Work out the finished part from the listing and answer in its coordinate system (mm). Face numbers are marked on the shaded views. A direction names the side the tool comes from. Round coordinates to 2 decimals unless told otherwise and drop trailing zeros. Order: outer loops, then holes, each group sorted by start corner. A loop starts at its lowest first (then second) coordinate and runs counter-clockwise, first axis right, second up. Notation, with made-up numbers: (30, -13.5) - (40, -13.5) arc R8 ccw to (40, 0.5) - close; hole circle Ø2 at (-18, 38). An arc over 180 degrees is marked (long way). One line per question, with ' | ' between items. Start each with the question number.
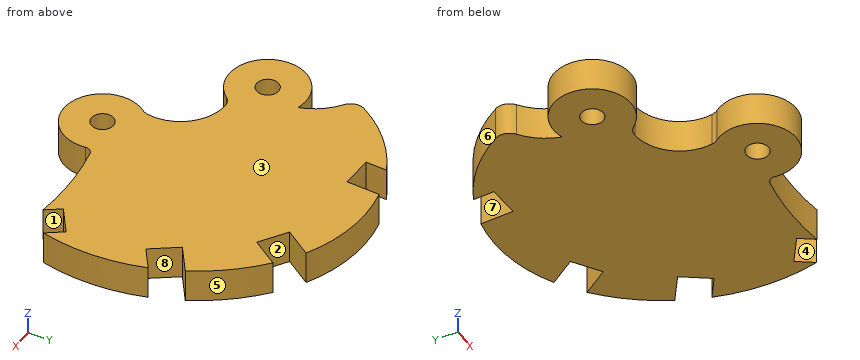
from build123d import *

# Parameters (mm, degrees)
SKETCH_1_R          = 1
EXTRUDE_1_DEPTH     = 3
CUT_EXTRUDE_1_DEPTH = 3
FILLET_3_R          = 0.635
FILLET_4_R          = 1.27
FILLET_5_R          = 1.27


with BuildPart() as part:
    # 스케치1 → 보스-돌출1 (new body)
    with BuildSketch(Plane.XY):
        with BuildLine():
            ThreePointArc((13.953884727, -10.4604054), (14.378598245, 0.342544853), (8.460782986, 9.390394228))
            ThreePointArc((8.460782986, 9.390394228), (-2.974719352, 12.059159282), (-12.129056489, 4.704491905))
            ThreePointArc((-12.129056489, 4.704491905), (-10.212753099, 3.28852822), (-9.098885827, 1.182234902))
            ThreePointArc((-9.098885827, 1.182234902), (-13.440703993, -3.372455138), (-7.178058569, -3.985528264))
            ThreePointArc((-7.178058569, -3.985528264), (-3.531014476, -5.328655626), (-2.617256463, -9.106216747))
            ThreePointArc((-2.617256463, -9.106216747), (-0.772979034, -14.843576338), (3.363017442, -10.4604054))
            ThreePointArc((3.363017442, -10.4604054), (8.658451084, -9.881913195), (13.953884727, -10.4604054))
        make_face()
        with Locations((-10.16, -2.153036707)):
            Circle(SKETCH_1_R, mode=Mode.SUBTRACT)
        with Locations((0, -11.43)):
            Circle(SKETCH_1_R, mode=Mode.SUBTRACT)
    extrude(amount=EXTRUDE_1_DEPTH)

    # 스케치2 → 컷-돌출1 (cut)
    with BuildSketch(Plane.XY.offset(3)):
        Polygon((12.294266072, -0.611273139), (10.692062425, 1.799944079), (13.190733117, 3.460258739), (14.792936764, 1.049041521), align=None)
        Polygon((-5.738219006, 9.252553702), (-2.846256152, 9.119979742), (-2.708873811, 12.11683244), (-5.600836664, 12.2494064), align=None)
        Polygon((4.882638145, 8.263381657), (7.266602202, 6.620901711), (8.96865396, 9.091330786), (6.584689903, 10.733810732), align=None)
        Polygon((11.087961457, -8.762836531), (13.499178676, -7.160632884), (15.159493336, -9.659303577), (12.748276117, -11.261507224), align=None)
    extrude(amount=-CUT_EXTRUDE_1_DEPTH, mode=Mode.SUBTRACT)

    # 필렛3
    fillet_3_edges = [part.edges().sort_by_distance(p)[0] for p in [
        (3.363017442, -10.4604054, 1.5),
    ]]
    fillet(fillet_3_edges, radius=FILLET_3_R)

    # 필렛4
    fillet_4_edges = [part.edges().sort_by_distance(p)[0] for p in [
        (-12.129056489, 4.704491905, 1.5),
    ]]
    fillet(fillet_4_edges, radius=FILLET_4_R)

    # 필렛5
    fillet_5_edges = [part.edges().sort_by_distance(p)[0] for p in [
        (-2.617256463, -9.106216747, 1.5),
        (-7.178058569, -3.985528264, 1.5),
    ]]
    fillet(fillet_5_edges, radius=FILLET_5_R)


solid = part.part
1) Section B-B on y = -11.43 is taken. Give the vertices of the cut face in (x, z), and give its area (3 significant figures).
2) For the marked faces 4, 5, 6, 7 and 8, determine the directions among +Z, -Z, +X, -X, +Y, -Y from which every point of the face is accessible in a straight line to the end or side of a thin tool.
3) Determine the mould class of the marked faces 1, 2 and 3 for opening direction X: released by +X, released by -X, zero draft, split by the parting line, or undercut.
4) Section C-C on x = -10.16 is taken. Give the vertices of the cut face in (y, z).
5) Section D-D on z = 1.1 is taken. Give the number of separate pieces and of enclosed holes in the cut face, and give its area (3 significant figures).
6) Straight lines are drawn through the part: line 1 (Y direction, x = -10.25, z = 2.35); line 2 (Y direction, x = -10.16, z = 1.1); line 3 (Y direction, x = 0, z = 0.95). For each, find the intervals that lie inside material, in ascending order.
7) Flat-ended cylindrical pins translate along their axes: pin 1 (1.5 mm diameter, centred on y = -3.5, z = 1, fed in from +X); pin 2 (1 mm diameter, centred on y = -11.5, z = 2.5, fed in from +X). Find the tip coordinate at first contact, or state that the pin passes through.
8) Section A-A on x = 0 is taken. Give the vertices of the cut face in (y, z), and give its area (3 significant figures).
Recorded:
1) outline: (-3.5, 0) - (-1, 0) - (-1, 3) - (-3.5, 3) - close; (1, 0) - (3.5, 0) - (3.5, 3) - (1, 3) - close | area: 15.0 mm²
2) face 4: +Z, -Z, -Y | face 5: +Z, -Z, +X, +Y | face 6: +Z, -Z, -X, +Y | face 7: +Z, -Z, +Y | face 8: +Z, -Z
3) face 1: released by +X | face 2: undercut | face 3: zero draft
4) outline: (-5.65, 0) - (-3.15, 0) - (-3.15, 3) - (-5.65, 3) - close; (-1.15, 0) - (1.35, 0) - (1.35, 3) - (-1.15, 3) - close; (3.23, 0) - (7.74, 0) - (7.74, 3) - (3.23, 3) - close
5) separate pieces: 1 | enclosed holes: 2 | area: 469 mm²
6) line 1: y = -5.65 to -3.15, -1.16 to 1.35, 3.33 to 7.63 | line 2: y = -5.65 to -3.15, -1.15 to 1.35, 3.23 to 7.74 | line 3: y = -14.93 to -12.43, -10.43 to 12.39
7) pin 1: stops at x = 15.02 | pin 2: stops at x = 3.5
8) outline: (-14.93, 0) - (-12.43, 0) - (-12.43, 3) - (-14.93, 3) - close; (-10.43, 0) - (12.39, 0) - (12.39, 3) - (-10.43, 3) - close | area: 76.0 mm²
